Geometry check sheet. Reference: the model listing, model coordinates, mm. Face numbers are marked on the shaded views. A direction names the side the tool comes from. Coordinates: 2 decimals unless noted, no trailing zeros. Write each loop counter-clockwise with the first axis right and the second up, starting at its lowest first coordinate (ties: lowest second). Pieces come first, ordered by that corner, then holes. Notation, with made-up numbers: (72.5, 16) -> (103.5, 16) arc R22 cw to (103.5, 47) -> close; hole circle Ø8 at (-37, -1). An arc over 180 degrees is marked (long way). Put each result on its own line as item: value. Start each with the question number.
from build123d import *

# Parameters (mm, degrees)
SKETCH1_R           = 98.425
SKETCH1_R_2         = 73.025
BOSS_EXTRUDE1_DEPTH = 20.32
SKETCH9_R           = 5.334
BOSS_EXTRUDE6_DEPTH = 27.94
CIRPATTERN5_COUNT   = 4


with BuildPart() as part:
    # Sketch1 → Boss-Extrude1 (new body)
    with BuildSketch(Plane(origin=(0, 0, 0), x_dir=(1, 0, 0), z_dir=(0, 1, 0))):
        Circle(SKETCH1_R)
        Circle(SKETCH1_R_2, mode=Mode.SUBTRACT)
    extrude(amount=BOSS_EXTRUDE1_DEPTH)

    # Sketch9 → Boss-Extrude6 (add)
    with BuildSketch(Plane(origin=(0, 20.32, 0), x_dir=(1, 0, 0), z_dir=(0, 1, 0))):
        with BuildLine():
            Line((-12.7, 85.725), (-12.7, 97.602206046))
            ThreePointArc((-12.7, 97.602206046), (0, 98.425), (12.7, 97.602206046))
            Line((12.7, 97.602206046), (12.7, 85.725))
            ThreePointArc((12.7, 85.725), (0, 73.025), (-12.7, 85.725))
        make_face()
        with Locations((0, 85.725)):
            Circle(SKETCH9_R, mode=Mode.SUBTRACT)
    boss_extrude6 = extrude(amount=BOSS_EXTRUDE6_DEPTH)

    # CirPattern5: Boss-Extrude6 ×4 about axis
    cirpattern5_axis = Axis((0, 0, 0), (0, 1, 0))
    for i in range(1, CIRPATTERN5_COUNT):
        add(boss_extrude6.rotate(cirpattern5_axis, i * 360 / CIRPATTERN5_COUNT))


solid = part.part
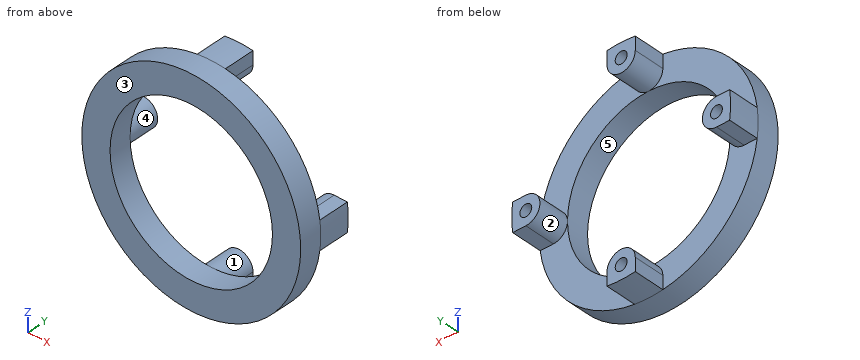
Item 1: Go/stop test with flat-tipped pins: P1, Ø9.5, axis at x = 91.5, y = 30, coming from the -Z side; P2, Ø1, axis at x = -52, y = 15, coming from the +Z side; P3, Ø1, axis at x = -51.5, y = 16, coming from the -Z side. Record where each tip stops, or that it passes through.
Item 2: Section check D-D, the plane y = 4. Enter the section's corners in (x, z) (3 decimals), and give its area (3 significant figures).
Item 3: Section check A-A, the plane y = 44. Enter the section's corners in (x, z) (3 decimals), and give its area (3 significant figures).
Item 4: Mould release check, pull along Z, two halves, no side actions. Record for the marked faces 1, 2 and 3: released by +Z, released by -Z, zero draft, split by the parting line, or undercut.
Item 5: Section check B-B, the plane z = -27. Enter the section's corners in (x, y).
Item 6: Access from +Z, -Z, +X, -X, +Y, -Y to the whole of each face (thin tool, end or side, straight path). Record for the marked faces 4 and 5.
Item 7: Section check C-C, the plane x = -48.5. Enter the section's corners in (y, z), and give its area (3 significant figures).
Item 8: Scan lines: line 1 along Z through (x, y) = (0, 37) (3 decimals); line 2 along Z through (x, y) = (1.5, 37.5). Record each from-to range of solid material in increasing order. Write a range as [from, to].
From the geometry:
1. P1: z = -12.7
1. P2: z = 83.88
1. P3: z = -84.18
2. outline: circle Ø196.85 at (0, 0); hole circle Ø146.05 at (0, 0)
2. area: 13,700 mm²
3. outline: (-97.602, -12.7) -> (-85.725, -12.7) arc R12.7 ccw to (-85.725, 12.7) -> (-97.602, 12.7) arc R98.425 ccw to start; (-12.7, -97.602) arc R98.425 ccw to (12.7, -97.602) -> (12.7, -85.725) arc R12.7 ccw to (-12.7, -85.725) -> close; (-12.7, 85.725) arc R12.7 ccw to (12.7, 85.725) -> (12.7, 97.602) arc R98.425 ccw to (-12.7, 97.602) -> close; (85.725, -12.7) -> (97.602, -12.7) arc R98.425 ccw to (97.602, 12.7) -> (85.725, 12.7) arc R12.7 ccw to start; hole circle Ø10.668 at (-85.725, 0); hole circle Ø10.668 at (0, -85.725); hole circle Ø10.668 at (0, 85.725); hole circle Ø10.668 at (85.725, 0)
3. area: 1,920 mm²
4. face 1: undercut
4. face 2: split by the parting line
4. face 3: zero draft
5. outline: (-94.65, 0) -> (-67.85, 0) -> (-67.85, 20.32) -> (-94.65, 20.32) -> close; (67.85, 0) -> (94.65, 0) -> (94.65, 20.32) -> (67.85, 20.32) -> close
6. face 4: +Y
6. face 5: +Y, -Y
7. outline: (0, -85.65) -> (20.32, -85.65) -> (20.32, -54.59) -> (0, -54.59) -> close; (0, 54.59) -> (20.32, 54.59) -> (20.32, 85.65) -> (0, 85.65) -> close
7. area: 1,260 mm²
8. line 1: [-98.425, -91.059], [-80.391, -73.025], [73.025, 80.391], [91.059, 98.425]
8. line 2: [-98.41, -90.84], [-80.61, -73.11], [73.11, 80.61], [90.84, 98.41]
